Check sheet for the drawn part. Datum: minimum x, y, z corner. Units: mm. Round coordinates to 2 decimals unless told otherwise and drop trailing zeros. Loops run counter-clockwise (first coordinate to the right, second up) from the corner with the lowest first, then second, coordinate; pieces in that order, holes last.
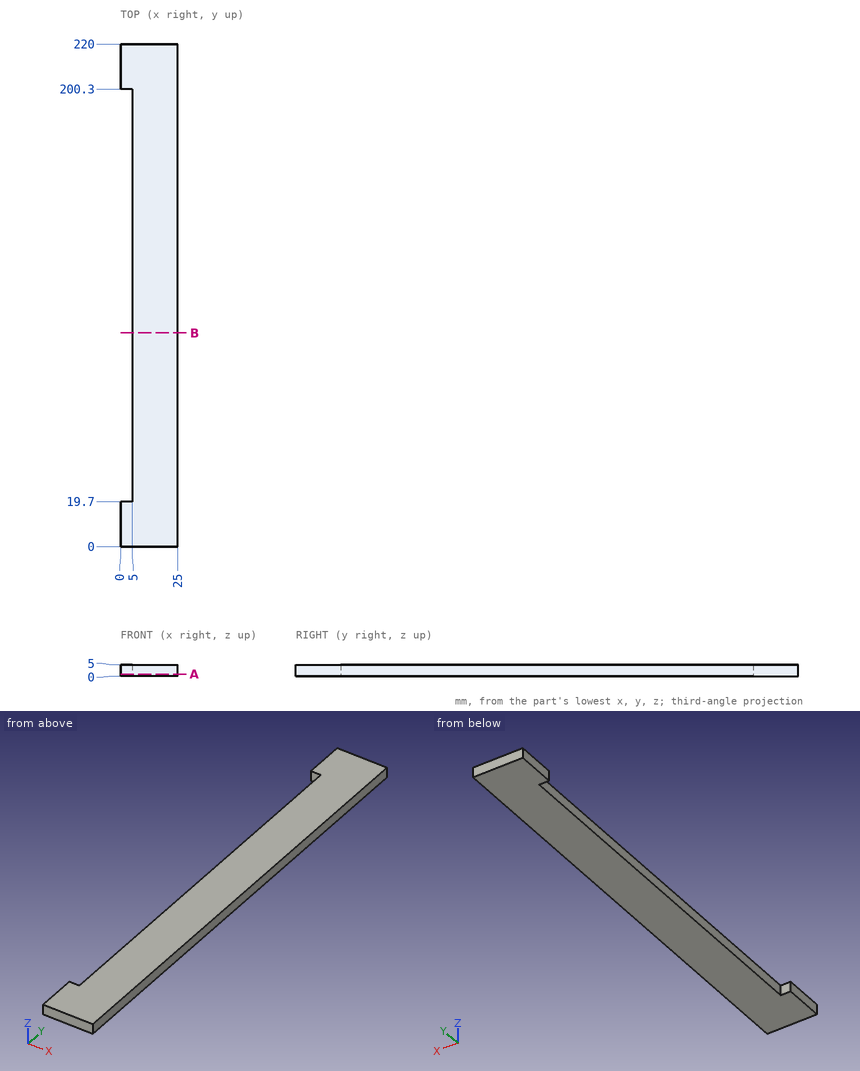
1. Gauge pin test, flat end, axial feed: P1, Ø3, axis at y = 183, z = 4.5, coming from the -X side. Record the tip position at first contact, or that the pin passes through.
2. Section check B-B (y = 93.5). Enter the section's corners in (x, z), then the cut area to 3 significant figures.
3. Scan lines: L1, parallel to Y at x = 4.25, z = 2.7; L2, parallel to X at y = 106.5, z = 0.7. Record each from-to range of solid material in increasing order.
4. Section check A-A (z = 0.8). Enter the section's corners in (x, y).
Taken from the geometry:
1. P1: stops at x = 5
2. outline: (5, 0) - (25, 0) - (25, 5) - (5, 5) - close
2. area: 100 mm2
3. L1: y = 0 to 19.7, 200.3 to 220
3. L2: x = 5 to 25
4. outline: (0, 0) - (25, 0) - (25, 220) - (0, 220) - (0, 200.3) - (5, 200.3) - (5, 19.7) - (0, 19.7) - close
